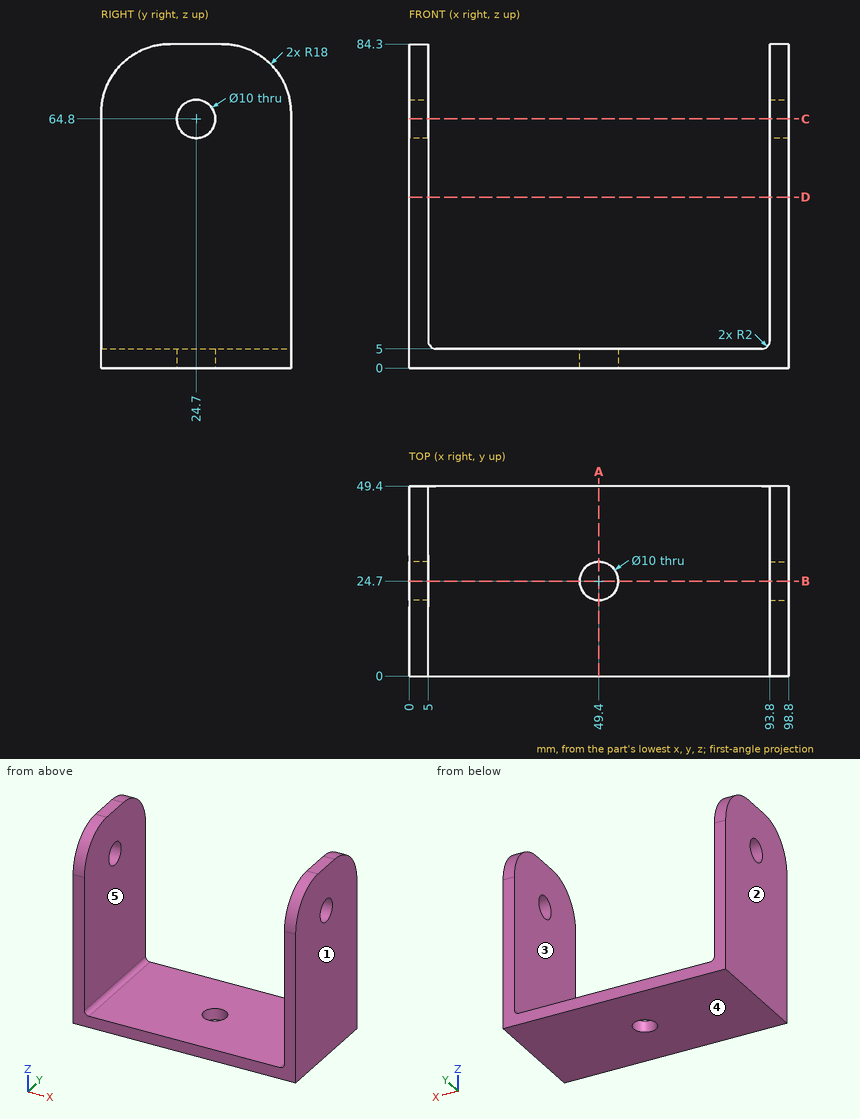
Check sheet for the drawn part. Datum: minimum x, y, z corner. Units: mm. A direction names the side the tool comes from. Give positions to 0.01 mm unless a question says otherwise; leave off trailing zeros. Write each loop counter-clockwise with the first axis right and the second up, starting at its lowest first coordinate (ties: lowest second). Pieces come first, ordered by that corner, then holes.
(1) Cross-section at C-C (z = 64.8). Enter the section's corners in (x, y).
(2) Material ranges on line 1 (X direction, y = 4, z = 32); line 2 (Y direction, x = 1.55, z = 64.8); line 3 (Z direction, x = 23, y = 30), recorded low to high.
(3) Access from +Z, -Z, +X, -X, +Y, -Y to the whole of each face (thin tool, end or side, straight path). Record for the marked faces 4 and 5.
(4) Gauge pin test, flat ends, axial feed: pin 1 (8 mm diameter, centred on x = 49.4, y = 24.7, fed in from +Z); pin 2 (1.5 mm diameter, centred on x = 75, y = 25, fed in from +Z). Record the tip position at first contact, or that the pin passes through.
(5) Cross-section at D-D (z = 44.5). Enter the section's corners in (x, y), plus the area to 3 significant figures.
(6) Cross-section at A-A (x = 49.4). Enter the section's corners in (y, z).
(7) Cross-section at B-B (y = 24.7). Enter the section's corners in (x, z).
(8) Mould release check, pull along X, two halves, no side actions. Record for the marked faces 1, 2 and 3: +X half, -X half, draft (parallel to the pull), parting line (faces both ways), or undercut.
Worked out:
1. outline: (0, 0) - (5, 0) - (5, 19.7) - (0, 19.7) - close; (0, 29.7) - (5, 29.7) - (5, 49.4) - (0, 49.4) - close; (93.8, 0) - (98.8, 0) - (98.8, 19.7) - (93.8, 19.7) - close; (93.8, 29.7) - (98.8, 29.7) - (98.8, 49.4) - (93.8, 49.4) - close
2. line 1: x = 0 to 5, 93.8 to 98.8
2. line 2: y = 0 to 19.7, 29.7 to 49.4
2. line 3: z = 0 to 5
3. face 4: -Z, +X, -X, +Y, -Y
3. face 5: +Z, +Y, -Y
4. pin 1: passes through
4. pin 2: stops at z = 5
5. outline: (0, 0) - (5, 0) - (5, 49.4) - (0, 49.4) - close; (93.8, 0) - (98.8, 0) - (98.8, 49.4) - (93.8, 49.4) - close
5. area: 494 mm2
6. outline: (0, 0) - (19.7, 0) - (19.7, 5) - (0, 5) - close; (29.7, 0) - (49.4, 0) - (49.4, 5) - (29.7, 5) - close
7. outline: (0, 0) - (44.4, 0) - (44.4, 5) - (7, 5) arc R2 cw to (5, 7) - (5, 59.8) - (0, 59.8) - close; (0, 69.8) - (5, 69.8) - (5, 84.3) - (0, 84.3) - close; (54.4, 0) - (98.8, 0) - (98.8, 59.8) - (93.8, 59.8) - (93.8, 7) arc R2 cw to (91.8, 5) - (54.4, 5) - close; (93.8, 69.8) - (98.8, 69.8) - (98.8, 84.3) - (93.8, 84.3) - close
8. face 1: +X half
8. face 2: -X half
8. face 3: undercut
